```python
from build123d import *

# Parameters (mm, degrees)
SKETCH_1_R          = 28.5
EXTRUDE_1_DEPTH     = 6
SKETCH_3_R          = 1.6
CUT_EXTRUDE_1_DEPTH = 16
SKETCH_4_R          = 1.6
CUT_EXTRUDE_2_DEPTH = 16
CUT_EXTRUDE_3_DEPTH = 10
FILLET_2_R          = 5
FILLET_3_R          = 4
SKETCH_7_R          = 7.5
SKETCH_7_R_2        = 12.5
CUT_EXTRUDE_5_DEPTH = 10
SKETCH_6_R          = 1.5
CUT_EXTRUDE_8_DEPTH = 10


with BuildPart() as part:
    # 草图1 → 凸台-拉伸1 (new body)
    with BuildSketch(Plane(origin=(0, 0, 0), x_dir=(1, 0, 0), z_dir=(0, 1, 0))):
        Circle(SKETCH_1_R)
        with BuildLine():
            Line((180, 28.5), (0, 28.5))
            ThreePointArc((0, 28.5), (20.152543264, 20.152543264), (28.5, 0))
            ThreePointArc((28.5, 0), (20.152543264, -20.152543264), (0, -28.5))
            Line((0, -28.5), (180, -28.5))
            ThreePointArc((180, -28.5), (151.5, 0), (180, 28.5))
        make_face()
        with Locations((180, 0)):
            Circle(SKETCH_1_R)
    extrude(amount=EXTRUDE_1_DEPTH)

    # 草图3 → 切除-拉伸1 (cut)
    with BuildSketch(Plane(origin=(0, 6, 0), x_dir=(1, 0, 0), z_dir=(0, 1, 0))):
        with Locations(Location((-13.5, 0, 0), (0, 0, 270))):
            Circle(SKETCH_3_R)
        with Locations(Location((-6.75, 11.691342951, 0), (0, 0, 270))):
            Circle(SKETCH_3_R)
        with Locations(Location((6.75, 11.691342951, 0), (0, 0, 270))):
            Circle(SKETCH_3_R)
        with Locations(Location((13.5, 0, 0), (0, 0, 270))):
            Circle(SKETCH_3_R)
        with Locations(Location((6.75, -11.691342951, 0), (0, 0, 270))):
            Circle(SKETCH_3_R)
        with Locations(Location((-6.75, -11.691342951, 0), (0, 0, 270))):
            Circle(SKETCH_3_R)
    extrude(amount=-CUT_EXTRUDE_1_DEPTH, mode=Mode.SUBTRACT)

    # 草图4 → 切除-拉伸2 (cut)
    with BuildSketch(Plane(origin=(0, 6, 0), x_dir=(1, 0, 0), z_dir=(0, 1, 0))):
        with Locations(Location((193.435028843, 13.435028843, 0), (0, 0, 270))):
            Circle(SKETCH_4_R)
        with Locations(Location((193.435028843, -13.435028843, 0), (0, 0, 270))):
            Circle(SKETCH_4_R)
        with Locations(Location((166.564971157, -13.435028843, 0), (0, 0, 270))):
            Circle(SKETCH_4_R)
        with Locations(Location((166.564971157, 13.435028843, 0), (0, 0, 270))):
            Circle(SKETCH_4_R)
    extrude(amount=-CUT_EXTRUDE_2_DEPTH, mode=Mode.SUBTRACT)

    # 草图5 → 切除-拉伸3 (cut)
    with BuildSketch(Plane(origin=(0, 6, 0), x_dir=(1, 0, 0), z_dir=(0, 1, 0))):
        Polygon((40, 0), (30.762395693, 16), (37.690598923, 20), (49.237604307, 0), (37.690598923, -20), (30.762395693, -16), align=None)
        Polygon((60, 0), (50.762395693, -16), (57.690598923, -20), (69.237604307, 0), (57.690598923, 20), (50.762395693, 16), align=None)
        Polygon((80, 0), (70.762395693, -16), (77.690598923, -20), (89.237604307, 0), (77.690598923, 20), (70.762395693, 16), align=None)
        Polygon((100, 0), (90.762395693, -16), (97.690598923, -20), (109.237604307, 0), (97.690598923, 20), (90.762395693, 16), align=None)
        Polygon((120, 0), (110.762395693, -16), (117.690598923, -20), (129.237604307, 0), (117.690598923, 20), (110.762395693, 16), align=None)
        Polygon((140, 0), (130.762395693, -16), (137.690598923, -20), (149.237604307, 0), (137.690598923, 20), (130.762395693, 16), align=None)
    extrude(amount=-CUT_EXTRUDE_3_DEPTH, mode=Mode.SUBTRACT)

    # 圆角2
    fillet_2_edges = [part.edges().sort_by_distance(p)[0] for p in [
        (40, 3, 0),
        (49.237604307, 3, 0),
        (120, 3, 0),
        (129.237604307, 3, 0),
        (140, 3, 0),
        (149.237604307, 3, 0),
        (60, 3, 0),
        (69.237604307, 3, 0),
        (80, 3, 0),
        (89.237604307, 3, 0),
        (100, 3, 0),
        (109.237604307, 3, 0),
    ]]
    fillet(fillet_2_edges, radius=FILLET_2_R)

    # 圆角3
    fillet_3_edges = [part.edges().sort_by_distance(p)[0] for p in [
        (117.690598923, 3, -20),
        (97.690598923, 3, -20),
        (77.690598923, 3, -20),
        (57.690598923, 3, -20),
        (110.762395693, 3, -16),
        (90.762395693, 3, -16),
        (70.762395693, 3, -16),
        (50.762395693, 3, -16),
        (110.762395693, 3, 16),
        (90.762395693, 3, 16),
        (70.762395693, 3, 16),
        (50.762395693, 3, 16),
        (117.690598923, 3, 20),
        (97.690598923, 3, 20),
        (77.690598923, 3, 20),
        (57.690598923, 3, 20),
        (37.690598923, 3, 20),
        (30.762395693, 3, 16),
        (30.762395693, 3, -16),
        (37.690598923, 3, -20),
        (137.690598923, 3, 20),
        (130.762395693, 3, 16),
        (137.690598923, 3, -20),
        (130.762395693, 3, -16),
    ]]
    fillet(fillet_3_edges, radius=FILLET_3_R - 0.0001)  # a hair under: the kernel refuses the full size

    # 草图7 → 切除-拉伸5 (cut)
    with BuildSketch(Plane(origin=(0, 6, 0), x_dir=(1, 0, 0), z_dir=(0, 1, 0))):
        with Locations(Location((0, 0, 0), (0, 0, 270))):
            Circle(SKETCH_7_R)
        with Locations(Location((180, 0, 0), (0, 0, 270))):
            Circle(SKETCH_7_R_2)
    extrude(amount=-CUT_EXTRUDE_5_DEPTH, mode=Mode.SUBTRACT)

    # 草图6 → 切除-拉伸8 (cut)
    with BuildSketch(Plane(origin=(0, 6, 0), x_dir=(1, 0, 0), z_dir=(0, 1, 0))):
        with Locations(Location((0, 24, 0), (0, 0, 270))):
            Circle(SKETCH_6_R)
        with Locations(Location((-24, 0, 0), (0, 0, 270))):
            Circle(SKETCH_6_R)
        with Locations(Location((0, -24, 0), (0, 0, 270))):
            Circle(SKETCH_6_R)
        with Locations(Location((180, 24, 0), (0, 0, 270))):
            Circle(SKETCH_6_R)
        with Locations(Location((204, 0, 0), (0, 0, 270))):
            Circle(SKETCH_6_R)
        with Locations(Location((180, -24, 0), (0, 0, 270))):
            Circle(SKETCH_6_R)
        with Locations(Location((45, -24, 0), (0, 0, 270))):
            Circle(SKETCH_6_R)
        with Locations(Location((45, 24, 0), (0, 0, 270))):
            Circle(SKETCH_6_R)
        with Locations(Location((90, -24, 0), (0, 0, 270))):
            Circle(SKETCH_6_R)
        with Locations(Location((90, 24, 0), (0, 0, 270))):
            Circle(SKETCH_6_R)
        with Locations(Location((135, -24, 0), (0, 0, 270))):
            Circle(SKETCH_6_R)
        with Locations(Location((135, 24, 0), (0, 0, 270))):
            Circle(SKETCH_6_R)
    extrude(amount=-CUT_EXTRUDE_8_DEPTH, mode=Mode.SUBTRACT)


solid = part.part
```
Geometry check sheet. Reference: the model listing, model coordinates, mm. A direction names the side the tool comes from. Round coordinates to 2 decimals unless told otherwise and drop trailing zeros. Write each question's results on one line, items separated by ' | '.
(1) Sectioned sample at A-A, the plane z = -4.5. Count the separate pieces of the cut face and the enclosed holes in it, plus the area to 3 significant figures.
Computed:
separate pieces: 9 | enclosed holes: 0 | area: 873 mm^2
(2) Draft check along X on faces 3 (the face through (77.22, 2.96, 18.41)), 4 (the face through (88, 6, 6)). Enter one of: pulls with the +X half, pulls with the -X half, needs draft (parallel to the pull), parting line crosses it, or undercut.
Computed:
face 3: undercut | face 4: needs draft
(3) Set-up check for faces 1 (the face through (137.22, 2.96, 18.41)), 2 (the face through (89, 3, 28.5)): record each of +Z, -Z, +X, -X, +Y, -Y from which the full face is reachable in a straight line by a thin tool's end or side.
Computed:
face 1: +Y, -Y | face 2: +Z, +X, -X, +Y, -Y
(4) Depth check by flat-ended pin: pin 1 Ø5 at (x, z) = (-13.5, 0) entering from +Y; pin 2 Ø1.8 at (x, z) = (180, 24) entering from -Y; pin 3 Ø2 at (y, z) = (3, 6.5) entering from -X; pin 4 Ø2 at (y, z) = (1.5, 3.5) entering from +X. Enter the tip coordinate at first touch or a pass-through.
Computed:
pin 1: stops at y = 6 | pin 2: passes through | pin 3: stops at x = -27.96 | pin 4: stops at x = 208.39
(5) Thickness scan on probe 1 along Z at (x, y) = (13, 2.5); probe 2 along X at (y, z) = (1, 23.5); probe 3 along X at (y, z) = (2.75, 25). Record the ranges inside material, lowest first. Write a range as from..to.
Computed:
probe 1: z = -28.5..-1.52, 1.52..28.5 | probe 2: x = -16.12..-1.41, 1.41..43.59, 46.41..88.59, 91.41..133.59, 136.41..178.59, 181.41..196.12 | probe 3: x = -13.68..-1.12, 1.12..43.88, 46.12..88.88, 91.12..133.88, 136.12..178.88, 181.12..193.68
